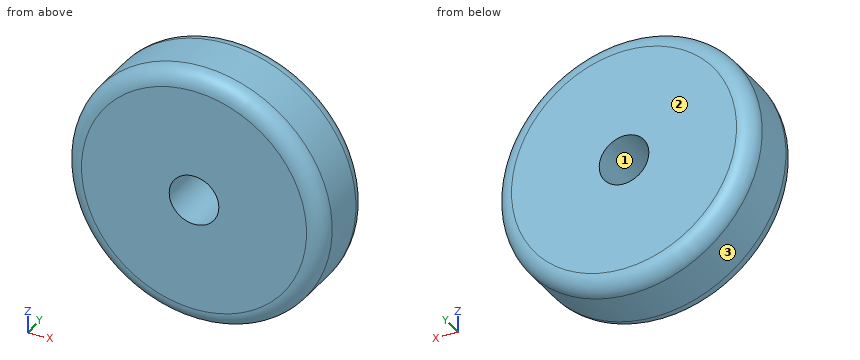
```python
from build123d import *

# Parameters (mm, degrees)
SKETCH1_R               = 39
BOSS_EXTRUDE1_DEPTH     = 11.5
FILLET1_R               = 5
CUT_EXTRUDE1_DEPTH      = 60.757844673
CUT_EXTRUDE1_DEPTH_BACK = 60.757844673
SKETCH2_R               = 7.5


with BuildPart() as part:
    # Sketch1 → Boss-Extrude1 (new, symmetric)
    with BuildSketch(Plane(origin=(0, 0, 0), x_dir=(1, 0, 0), z_dir=(0, 1, 0))):
        with Locations(Location((0, 0, 0), (0, 0, 270))):
            Circle(SKETCH1_R)
    extrude(amount=BOSS_EXTRUDE1_DEPTH, both=True)

    # Fillet1
    fillet1_edges = [part.edges().sort_by_distance(p)[0] for p in [
        (0, -11.5, -39),
        (0, 11.5, -39),
    ]]
    fillet(fillet1_edges, radius=FILLET1_R)

    # Sketch2 → Cut-Extrude1 (cut, two sides: drawn at the far end of the back side and taken through both)
    with BuildSketch(Plane(origin=(0, 11.5, 0), x_dir=(1, 0, 0), z_dir=(0, 1, 0)).offset(-CUT_EXTRUDE1_DEPTH_BACK)):
        with Locations(Location((0, 0, 0), (0, 0, 270))):
            Circle(SKETCH2_R)
    extrude(amount=CUT_EXTRUDE1_DEPTH + CUT_EXTRUDE1_DEPTH_BACK, mode=Mode.SUBTRACT)


solid = part.part
```
Geometry: final body of the model. Coordinates: model frame, mm. Face numbers are marked on the shaded views. Coordinates: 2 decimals unless noted, no trailing zeros. Order: outer loops, then holes, each group sorted by start corner. A loop starts at its lowest first (then second) coordinate and runs counter-clockwise, first axis right, second up. Notation, with made-up numbers: (14.25, 7.5) -> (52.25, 7.5) arc R22 ccw to (52.25, 24.5) -> close; hole circle Ø2 at (39, -7.5). An arc over 180 degrees is marked (long way). Write item = value, one per line.
(1) Pin query (flat end, axial travel): pin 1 Ø6 at (y, z) = (-1.5, 24.5) entering from -X; pin 2 Ø5 at (y, z) = (-3, 21.5) entering from +X; pin 3 Ø2 at (x, z) = (23.5, -28.5) entering from -Y; pin 4 Ø9 at (x, z) = (0, 0) entering from +Y. Return the tip coordinate at first contact, or that it passes through.
Solved:
pin_1 = -32.54
pin_2 = 34.06
pin_3 = -11.11
pin_4 = through
(2) Cut plane A-A on x = 0. Return loops of the section in (y, z).
Solved:
outline = (-11.5, -34) arc R5 ccw to (-6.5, -39) -> (6.5, -39) arc R5 ccw to (11.5, -34) -> (11.5, -7.5) -> (-11.5, -7.5) -> close; (-11.5, 7.5) -> (11.5, 7.5) -> (11.5, 34) arc R5 ccw to (6.5, 39) -> (-6.5, 39) arc R5 ccw to (-11.5, 34) -> close
(3) Line query: line 1 (X direction, y = -4, z = 0); line 2 (Z direction, x = 2, y = 6.5); line 3 (Z direction, x = -30, y = -7). Output: solid intervals per line, ascending.
Solved:
line_1 = -39 to -7.5, 7.5 to 39
line_2 = -38.95 to -7.23, 7.23 to 38.95
line_3 = -24.88 to 24.88
(4) Cut plane B-B on z = 0. Return loops of the section in (x, y), plus the area to 3 significant figures.
Solved:
outline = (-39, -6.5) arc R5 ccw to (-34, -11.5) -> (-7.5, -11.5) -> (-7.5, 11.5) -> (-34, 11.5) arc R5 ccw to (-39, 6.5) -> close; (7.5, -11.5) -> (34, -11.5) arc R5 ccw to (39, -6.5) -> (39, 6.5) arc R5 ccw to (34, 11.5) -> (7.5, 11.5) -> close
area = 1,430 mm²
(5) Pull-direction query (X, two-part tool) for the marked faces 1, 2 and 3; classes: pulls with the +X half, pulls with the -X half, needs draft (parallel to the pull), parting line crosses it, or undercut.
Solved:
face_1 = undercut
face_2 = needs draft
face_3 = parting line crosses it
